Source: CAD feature listing. Evaluate the final solid. Frame: model axes, mm. Face numbers are marked on the shaded views. A direction names the side the tool comes from. Coordinates: 2 decimals unless noted, no trailing zeros. Order: outer loops, then holes, each group sorted by start corner. A loop starts at its lowest first (then second) coordinate and runs counter-clockwise, first axis right, second up. Notation, with made-up numbers: (29.25, 75.5) -> (66.25, 75.5) arc R15 cw to (66.25, 85.5) -> close; hole circle Ø7 at (-19.75, 27). An arc over 180 degrees is marked (long way). Put each result on its own line as item: value.
from build123d import *

# Parameters (mm, degrees)
SKETCH1_W           = 146
SKETCH1_H           = 50
BOSS_EXTRUDE1_DEPTH = 10
SKETCH2_R           = 3.175
CUT_EXTRUDE1_DEPTH  = 10
SKETCH3_W           = 12
SKETCH3_H           = 50
BOSS_EXTRUDE2_DEPTH = 38
SKETCH4_R           = 2.2
BOSS_EXTRUDE3_DEPTH = 82
SKETCH5_W           = 70
SKETCH5_H           = 17
BOSS_EXTRUDE4_DEPTH = 5.5
SKETCH6_W           = 70
SKETCH6_H           = 10.2
CUT_EXTRUDE2_DEPTH  = 3.2


with BuildPart() as part:
    # Sketch1 → Boss-Extrude1 (new body)
    with BuildSketch(Plane(origin=(0, 0, 0), x_dir=(1, 0, 0), z_dir=(0, 1, 0))):
        with Locations((73, -25)):
            Rectangle(SKETCH1_W, SKETCH1_H)
    extrude(amount=BOSS_EXTRUDE1_DEPTH)

    # Sketch2 → Cut-Extrude1 (cut)
    with BuildSketch(Plane(origin=(0, 10, 0), x_dir=(1, 0, 0), z_dir=(0, 1, 0))):
        with Locations((9.5, -12.3)):
            Circle(SKETCH2_R)
        with Locations((10.5, -37.680307327)):
            Circle(SKETCH2_R)
    cut_extrude1 = extrude(amount=-CUT_EXTRUDE1_DEPTH, mode=Mode.SUBTRACT)

    # Mirror1: Cut-Extrude1 across plane
    add(cut_extrude1.mirror(Plane.ZY.offset(-73)), mode=Mode.SUBTRACT)

    # Sketch3 → Boss-Extrude2 (add)
    with BuildSketch(Plane(origin=(0, 10, 0), x_dir=(1, 0, 0), z_dir=(0, 1, 0))):
        with Locations((115, -25)):
            Rectangle(SKETCH3_W, SKETCH3_H)
        with Locations((33, -25)):
            Rectangle(SKETCH3_W, SKETCH3_H)
    extrude(amount=BOSS_EXTRUDE2_DEPTH)

    # Sketch4 → Boss-Extrude3 (add)
    with BuildSketch(Plane(origin=(121, 0, 0), x_dir=(0, 0, -1), z_dir=(1, 0, 0))):
        with Locations((-25, 30.2)):
            Circle(SKETCH4_R)
    extrude(amount=-BOSS_EXTRUDE3_DEPTH)

    # Sketch5 → Boss-Extrude4 (add)
    with BuildSketch(Plane(origin=(0, 10, 0), x_dir=(1, 0, 0), z_dir=(0, 1, 0))):
        with Locations((74, -25)):
            Rectangle(SKETCH5_W, SKETCH5_H)
    extrude(amount=BOSS_EXTRUDE4_DEPTH)

    # Sketch6 → Cut-Extrude2 (cut)
    with BuildSketch(Plane(origin=(0, 15.5, 0), x_dir=(1, 0, 0), z_dir=(0, 1, 0))):
        with Locations((74, -25)):
            Rectangle(SKETCH6_W, SKETCH6_H)
    extrude(amount=-CUT_EXTRUDE2_DEPTH, mode=Mode.SUBTRACT)


solid = part.part
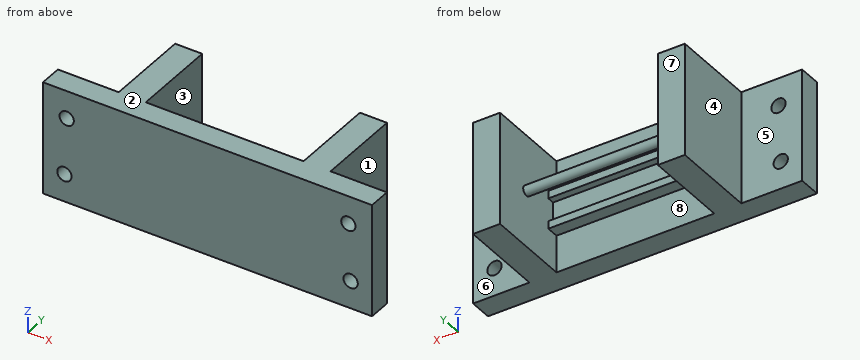
1. Cut plane D-D on z = 25. Output: boundary loops of the cut face in (x, y), plus the area to 3 significant figures.
Numbers:
outline: (0, 0) -> (146, 0) -> (146, 10) -> (121, 10) -> (121, 48) -> (109, 48) -> (109, 32.4) -> (39, 32.4) -> (39, 48) -> (27, 48) -> (27, 10) -> (0, 10) -> close; hole (39, 12.3) -> (109, 12.3) -> (109, 28) -> (39, 28) -> close
area: 2,840 mm2
2. First-contact query: pin 1 (8 mm diameter, centred on x = 75, z = 6.5, fed in from +Y); pin 2 (3 mm diameter, centred on x = 107, y = 37, fed in from +Z); pin 3 (1 mm diameter, centred on x = 69.5, y = 14, fed in from -Z); pin 4 (19 mm diameter, centred on y = 21.5, z = 26, fed in from -X). Flat tips, straight axial feed; report the tip coordinate or a pass-through.
Numbers:
pin 1: stops at y = 10
pin 2: passes through
pin 3: stops at z = 16.5
pin 4: stops at x = 27
3. Cut plane B-B on x = 79.5. Output: boundary loops of the cut face in (y, z).
Numbers:
outline: (0, 0) -> (10, 0) -> (10, 16.5) -> (15.5, 16.5) -> (15.5, 19.9) -> (12.3, 19.9) -> (12.3, 30.1) -> (15.5, 30.1) -> (15.5, 33.5) -> (10, 33.5) -> (10, 50) -> (0, 50) -> close; circle Ø4.4 at (30.2, 25)
4. Ray query, line 1 along X through (y, z) = (5, 12); line 2 along X through (y, z) = (14, 21); line 3 along Z through (x, y) = (136.5, 5) (3 decimals). Return the intervals inside material, ascending.
Numbers:
line 1: x = 0 to 6.34, 12.66 to 133.34, 139.66 to 146
line 2: x = 27 to 39, 109 to 121
line 3: z = 0 to 9.125, 15.475 to 34.667, 40.694 to 50
5. Cut plane A-A on z = 12.3. Output: boundary loops of the cut face in (x, y) (3 decimals).
Numbers:
outline: (0, 0) -> (6.325, 0) -> (6.325, 10) -> (0, 10) -> close; (12.675, 0) -> (133.325, 0) -> (133.325, 10) -> (121, 10) -> (121, 48) -> (109, 48) -> (109, 10) -> (39, 10) -> (39, 48) -> (27, 48) -> (27, 10) -> (12.675, 10) -> close; (139.675, 0) -> (146, 0) -> (146, 10) -> (139.675, 10) -> close
6. Set-up query: the marked faces 5, 6, 7 and 8. Return all of +Z, -Z, +X, -X, +Y, -Y with unobstructed straight access to the full face (end or side cutting, diameter ignored); none if empty.
Numbers:
face 5: +Z, -Z, -X, +Y
face 6: +Z, -Z, +X, +Y
face 7: +Z, -Z, +X, -X, +Y
face 8: -Z, +Y
7. Pull-direction query (X, two-part tool) for the marked faces 1, 2, 3 and 4; classes: pulls with the +X half, pulls with the -X half, needs draft (parallel to the pull), parting line crosses it, or undercut.
Numbers:
face 1: pulls with the +X half
face 2: needs draft
face 3: undercut
face 4: pulls with the -X half
8. Cut plane C-C on y = 19. Output: boundary loops of the cut face in (x, z), plus the area to 3 significant figures.
Numbers:
outline: (27, 0) -> (39, 0) -> (39, 50) -> (27, 50) -> close; (109, 0) -> (121, 0) -> (121, 50) -> (109, 50) -> close
area: 1,200 mm2
